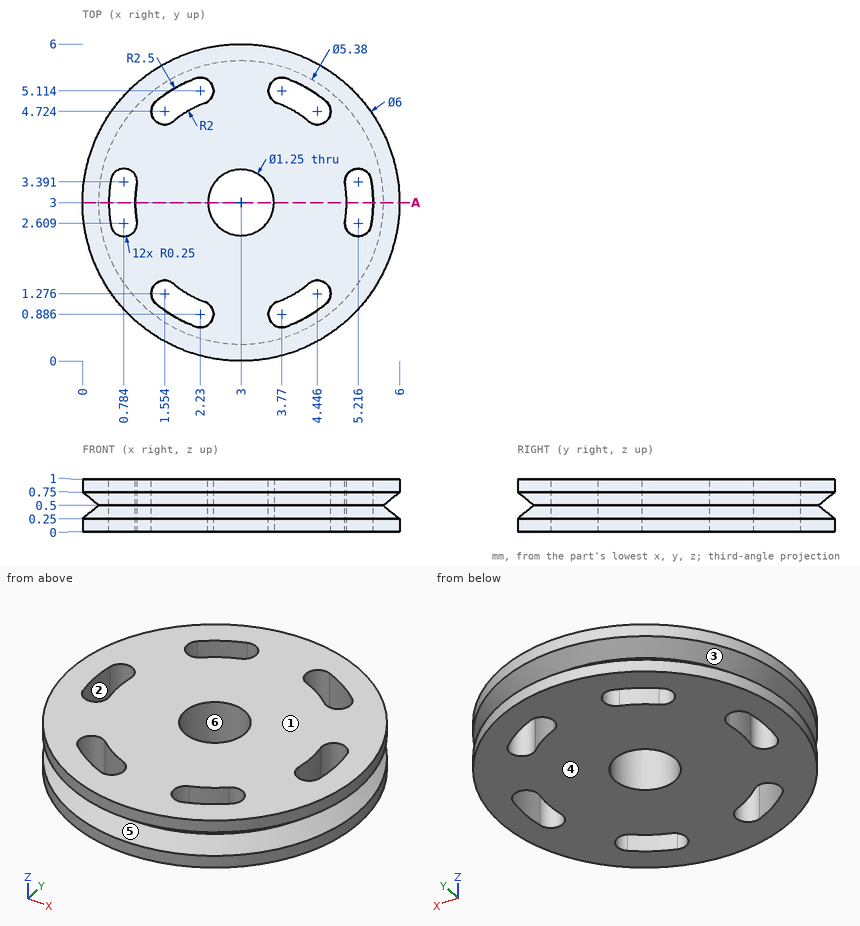
Here's the drawing with two shaded views (mm, measured from the low corner). I have some questions. A direction names the side the tool comes from. Give positions to 0.01 mm unless a question says otherwise; leave off trailing zeros.
Q1. We'd pull the mould along Z, two halves only. Please class the marked faces 4, 5 and 6: +Z half, -Z half, draft (parallel to the pull), parting line (faces both ways), or undercut.
Q2. Suppose I cut it at A-A, the plane y = 3. Count the separate pieces of the cut face and the enclosed holes in it.
Q3. If I drill on line 1 along X through (y, z) = (2.95, 0.95); line 2 along X through (y, z) = (2.85, 0.4) (1 decimal); line 3 along Y through (x, z) = (1.95, 0.45) (1 decimal), over which ranges is the centre line in solid material (lowest first)?
Q4. For the marked faces 1, 2 and 3, which set-ups out of +Z, -Z, +X, -X, +Y, -Y let a thin tool reach every point of the face, with its end or its side?
Solution:
1. face 4: -Z half
1. face 5: undercut
1. face 6: draft
2. separate pieces: 4
2. enclosed holes: 0
3. line 1: x = 0 to 0.5, 1 to 2.38, 3.62 to 5, 5.5 to 6
3. line 2: x = 0.2 to 0.5, 1 to 2.4, 3.6 to 5, 5.5 to 5.8
3. line 3: y = 0.5 to 0.7, 1.3 to 4.7, 5.3 to 5.5
4. face 1: +Z, +X, -X, +Y, -Y
4. face 2: +Z, -Z
4. face 3: none
